Source: CAD feature listing. Evaluate the final solid. Frame: model axes, mm. Face numbers are marked on the shaded views. Coordinates: 2 decimals unless noted, no trailing zeros. Write each loop counter-clockwise with the first axis right and the second up, starting at its lowest first coordinate (ties: lowest second). Pieces come first, ordered by that corner, then holes. Notation, with made-up numbers: (-24.75, -17) - (25.25, -17) arc R13 ccw to (25.25, -10) - close; hole circle Ø5 at (77, -23). An arc over 180 degrees is marked (long way). One line per question, with ' | ' between items.
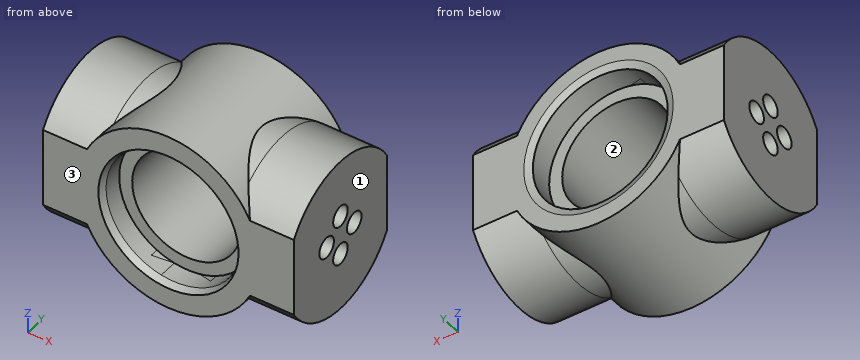
from build123d import *
from OCP.BRepFilletAPI import BRepFilletAPI_MakeChamfer
from build123d.topology import SkipClean

# Parameters (mm, degrees)
SKIZZE1_R                            = 25
SKIZZE1_R_2                          = 18.6
AUFSATZ_LINEAR_AUSTRAGEN1_DEPTH      = 18.5
SKIZZE2_R                            = 18.6
SKIZZE2_R_2                          = 15
AUFSATZ_LINEAR_AUSTRAGEN2_DEPTH      = 11.3
SKIZZE3_R                            = 21.5
AUFSATZ_LINEAR_AUSTRAGEN3_DEPTH      = 16
SKIZZE4_R                            = 2.9
SCHNITT_LINEAR_AUSTRAGEN1_DEPTH      = 9.1
SKIZZE5_OUTSIDE_W                    = 64.118
SKIZZE5_OUTSIDE_H                    = 71.118
SKIZZE5_OUTSIDE_W_2                  = 37
SKIZZE5_OUTSIDE_H_2                  = 50
SCHNITT_LINEAR_AUSTRAGEN2_DEPTH      = 67.342867843
SCHNITT_LINEAR_AUSTRAGEN2_DEPTH_BACK = 67.342867843
AUFSATZ_LINEAR_AUSTRAGEN4_DEPTH      = 37.2
SKIZZE8_R                            = 18.6
SCHNITT_LINEAR_AUSTRAGEN3_DEPTH      = 53.059581422
FASE1_SIZE                           = 2
FASE1_SIZE2                          = 0.727940469


with BuildPart() as part:
    # Skizze1 → Aufsatz-Linear austragen1 (new, symmetric)
    with BuildSketch(Plane(origin=(0, 0, 0), x_dir=(1, 0, 0), z_dir=(0, 1, 0))):
        with Locations(Location((0, 0, 0), (0, 0, 270))):
            Circle(SKIZZE1_R)
        with Locations(Location((0, 0, 0), (0, 0, 270))):
            Circle(SKIZZE1_R_2, mode=Mode.SUBTRACT)
    extrude(amount=AUFSATZ_LINEAR_AUSTRAGEN1_DEPTH, both=True)

    # Skizze2 → Aufsatz-Linear austragen2 (add, symmetric)
    with BuildSketch(Plane(origin=(0, 0, 0), x_dir=(1, 0, 0), z_dir=(0, 1, 0))):
        with Locations(Location((0, 0, 0), (0, 0, 270))):
            Circle(SKIZZE2_R)
        with Locations(Location((0, 0, 0), (0, 0, 270))):
            Circle(SKIZZE2_R_2, mode=Mode.SUBTRACT)
    extrude(amount=AUFSATZ_LINEAR_AUSTRAGEN2_DEPTH, both=True)

    # Skizze3 → Aufsatz-Linear austragen3 (add)
    with BuildSketch(Plane(origin=(18.6, 0, 0), x_dir=(0, 0, -1), z_dir=(1, 0, 0))):
        with Locations(Location((0, 0, 0), (0, 0, 140.982439232))):
            Circle(SKIZZE3_R)
    aufsatz_linear_austragen3 = extrude(amount=AUFSATZ_LINEAR_AUSTRAGEN3_DEPTH)

    # Skizze4 → Schnitt-Linear austragen1 (cut)
    with BuildSketch(Plane(origin=(34.6, 0, 0), x_dir=(0, 0, -1), z_dir=(1, 0, 0))):
        with Locations((-5.5, 0)):
            Circle(SKIZZE4_R)
        with Locations((0, 5.5)):
            Circle(SKIZZE4_R)
        with Locations((5.5, 0)):
            Circle(SKIZZE4_R)
        with Locations((0, -5.5)):
            Circle(SKIZZE4_R)
    schnitt_linear_austragen1 = extrude(amount=-SCHNITT_LINEAR_AUSTRAGEN1_DEPTH, mode=Mode.SUBTRACT)

    # Spiegeln1: Aufsatz-Linear austragen3, Schnitt-Linear austragen1 across plane
    add(aufsatz_linear_austragen3.mirror(Plane(origin=(0, 0, 0), x_dir=(0, 0, 1), z_dir=(1, 0, 0))))
    add(schnitt_linear_austragen1.mirror(Plane(origin=(0, 0, 0), x_dir=(0, 0, 1), z_dir=(1, 0, 0))), mode=Mode.SUBTRACT)

    # Skizze5 outside → Schnitt-Linear austragen2 (cut, two sides)
    with BuildSketch(Plane(origin=(0, 29.28598322, 0), x_dir=(0, -1, 0), z_dir=(-1, 0, 0))) as schnitt_linear_austragen2_sk:
        with Locations((29.286, 0)):
            Rectangle(SKIZZE5_OUTSIDE_W, SKIZZE5_OUTSIDE_H)
        with Locations((29.28598322, 0)):
            Rectangle(SKIZZE5_OUTSIDE_W_2, SKIZZE5_OUTSIDE_H_2, mode=Mode.SUBTRACT)
    extrude(amount=SCHNITT_LINEAR_AUSTRAGEN2_DEPTH, mode=Mode.SUBTRACT)
    extrude(schnitt_linear_austragen2_sk.sketch, amount=-SCHNITT_LINEAR_AUSTRAGEN2_DEPTH_BACK, mode=Mode.SUBTRACT)

    # Skizze7 → Aufsatz-Linear austragen4 (add)
    with BuildSketch(Plane.ZY.offset(-18.6)):
        with BuildLine():
            Line((16.704490414, 13.535508856), (16.704490414, -13.535508856))
            ThreePointArc((16.704490414, -13.535508856), (21.5, 0), (16.704490414, 13.535508856))
        make_face()
    aufsatz_linear_austragen4 = extrude(amount=AUFSATZ_LINEAR_AUSTRAGEN4_DEPTH)

    # Spiegeln2: Aufsatz-Linear austragen4 across plane
    add(aufsatz_linear_austragen4.mirror(Plane.XY))

    # Skizze8 → Schnitt-Linear austragen3 (cut, through all)
    with BuildSketch(Plane(origin=(0, 11.3, 0), x_dir=(1, 0, 0), z_dir=(0, 1, 0))):
        with Locations(Location((0, 0, 0), (0, 0, 100.458673289))):
            Circle(SKIZZE8_R)
    schnitt_linear_austragen3 = extrude(amount=SCHNITT_LINEAR_AUSTRAGEN3_DEPTH, mode=Mode.SUBTRACT)

    # Spiegeln3: Schnitt-Linear austragen3 across plane
    with SkipClean():  # the faces are left unmerged after this step: merging them gives an invalid solid
        add(schnitt_linear_austragen3.mirror(Plane.ZX), mode=Mode.SUBTRACT)

    # Fase1: one chamfer whose edges measure the first distance from different faces: ONE call of the kernel's chamfer builder (chamfer() names one face for all edges)
    fase1_edges_1 = [part.edges().sort_by_distance(p)[0] for p in [
        (18.522584239, -18.5, -1.695250166),
    ]]
    fase1_side_1 = [part.faces().sort_by_distance(p)[0] for p in [
        (18.522584239, -14.9, -1.695250166),
    ]]
    fase1_edges_2 = [part.edges().sort_by_distance(p)[0] for p in [
        (0, 18.5, -18.6),
    ]]
    fase1_side_2 = [part.faces().sort_by_distance(p)[0] for p in [
        (0, 18.5, 24.146264678),
    ]]
    fase1 = BRepFilletAPI_MakeChamfer(part.part.solid().wrapped)
    for e in fase1_edges_1:
        fase1.Add(FASE1_SIZE, FASE1_SIZE2, e.wrapped, fase1_side_1[0].wrapped)  # the first distance lies on this face
    for e in fase1_edges_2:
        fase1.Add(FASE1_SIZE, FASE1_SIZE2, e.wrapped, fase1_side_2[0].wrapped)  # the first distance lies on this face
    add(Compound.cast(fase1.Shape()), mode=Mode.REPLACE)


solid = part.part
Item 1: Cut plane B-B on y = 5.5. Return loops of the section in (x, z).
Check sheet entries:
outline: (-34.6, -20.78) - (-13.89, -20.78) arc R25 ccw to (13.89, -20.78) - (34.6, -20.78) - (34.6, -2.9) - (25.5, -2.9) - (25.5, 2.9) - (34.6, 2.9) - (34.6, 20.78) - (13.89, 20.78) arc R25 ccw to (-13.89, 20.78) - (-34.6, 20.78) - (-34.6, 2.9) - (-25.5, 2.9) - (-25.5, -2.9) - (-34.6, -2.9) - close; hole circle Ø30 at (0, 0)
Item 2: Cut plane C-C on y = 16. Return loops of the section in (x, z).
Check sheet entries:
outline: (-34.6, -14.36) - (-20.46, -14.36) arc R25 ccw to (20.46, -14.36) - (34.6, -14.36) - (34.6, 14.36) - (20.46, 14.36) arc R25 ccw to (-20.46, 14.36) - (-34.6, 14.36) - close; hole circle Ø37.2 at (0, 0)
Item 3: Cut plane A-A on y = 0. Return loops of the section in (x, z), and give its area (3 significant figures).
Check sheet entries:
outline: (-34.6, -21.5) - (-12.76, -21.5) arc R25 ccw to (12.76, -21.5) - (34.6, -21.5) - (34.6, -8.4) - (25.5, -8.4) - (25.5, -2.6) - (34.6, -2.6) - (34.6, 2.6) - (25.5, 2.6) - (25.5, 8.4) - (34.6, 8.4) - (34.6, 21.5) - (12.76, 21.5) arc R25 ccw to (-12.76, 21.5) - (-34.6, 21.5) - (-34.6, 8.4) - (-25.5, 8.4) - (-25.5, 2.6) - (-34.6, 2.6) - (-34.6, -2.6) - (-25.5, -2.6) - (-25.5, -8.4) - (-34.6, -8.4) - close; hole circle Ø30 at (0, 0) | area: 2,180 mm²
Item 4: Ray query, line 1 along Y through (x, z) = (29.25, 0); line 2 along Z through (x, y) = (0, -14); line 3 along X through (y, z) = (-10, 0.5). Return the intervals inside material, ascending. Write a range as [from, to].
Check sheet entries:
line 1: [-18.5, -8.4], [-2.6, 2.6], [8.4, 18.5] | line 2: [-25, -18.6], [18.6, 25] | line 3: [-34.6, -14.99], [14.99, 34.6]
Item 5: Mould query, pull axis X, two halves, no side actions, for the marked faces 1, 2 and 3. Classes: pulls with the +X half, pulls with the -X half, needs draft (parallel to the pull), parting line crosses it, or undercut.
Check sheet entries:
face 1: pulls with the +X half | face 2: undercut | face 3: needs draft
Item 6: Pin query (flat end, axial travel): pin 1 Ø3 at (y, z) = (-5.5, 0.5) entering from +X; pin 2 Ø6.5 at (y, z) = (-5.5, 0) entering from -X; pin 3 Ø12 at (x, y) = (-27, 11.5) entering from +Z; pin 4 Ø1.5 at (x, y) = (21, -11.5) entering from -Z. Return the tip coordinate at first contact, or that it passes through.
Check sheet entries:
pin 1: x = 25.5 | pin 2: x = -34.6 | pin 3: z = 20.78 | pin 4: z = -18.62
